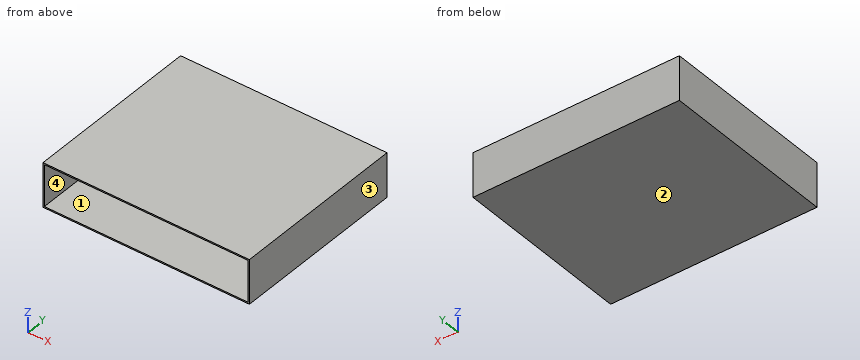
```python
from build123d import *

# Parameters (mm, degrees)
F0_W     = 900
F0_H     = 225
F1_DEPTH = 1050
F2_T     = -7


with BuildPart() as f1:
    # F0 (on Right) → F1 (new body)
    with BuildSketch(Plane.YZ):
        with Locations((450, -112.5)):
            Rectangle(F0_W, F0_H)
    extrude(amount=-F1_DEPTH)

    # F2
    f2_openings = [f1.faces().sort_by_distance(p)[0] for p in [
        (-525, 0, -112.5),
    ]]
    offset(amount=F2_T, openings=f2_openings)


solid = f1.part
```
CAD build for the part. Positions are in the model's coordinates, mm. Face numbers are marked on the shaded views. Round coordinates to 2 decimals unless told otherwise and drop trailing zeros. Order: outer loops, then holes, each group sorted by start corner. A loop starts at its lowest first (then second) coordinate and runs counter-clockwise, first axis right, second up.
Q1. Two-plate mould, pull along X, no slides. Class the marked faces 1, 2, 3 and 4: pulls with the +X half, pulls with the -X half, needs draft (parallel to the pull), parting line crosses it, or undercut.
Q2. Drop a flat-ended pin along its axis: pin 1 (2 mm diameter, centred on x = -882, z = -71.5, fed in from -Y). Give the stop position or say it passes through.
Q3. Wall check: L1, parallel to X at y = 696, z = -127.5; L2, parallel to Z at x = -298, y = 863; L3, parallel to Y at x = -479.5, z = -89.5. Give the ranges that are in metal, low to high.
Q4. Slice it at B-B (x = -311.5). Write the cut outline in (y, z).
Q5. Slice it at A-A (y = 579.5). Write the cut outline in (x, z).
Q6. Slice it at C-C (z = -193.5). Write the cut outline in (x, y).
Results below:
1. face 1: undercut
1. face 2: needs draft
1. face 3: pulls with the +X half
1. face 4: undercut
2. pin 1: stops at y = 893
3. L1: x = -1050 to -1043, -7 to 0
3. L2: z = -225 to -218, -7 to 0
3. L3: y = 893 to 900
4. outline: (0, -225) - (900, -225) - (900, 0) - (0, 0) - (0, -7) - (893, -7) - (893, -218) - (0, -218) - close
5. outline: (-1050, -225) - (0, -225) - (0, 0) - (-1050, 0) - close; hole (-1043, -218) - (-7, -218) - (-7, -7) - (-1043, -7) - close
6. outline: (-1050, 0) - (-1043, 0) - (-1043, 893) - (-7, 893) - (-7, 0) - (0, 0) - (0, 900) - (-1050, 900) - close
